from build123d import *

# Parameters (mm, degrees)
SKETCH1_R               = 12.7
BOSS_EXTRUDE1_DEPTH     = 0.79375
SKETCH2_R               = 9.525
BOSS_EXTRUDE2_DEPTH     = 6.35
SKETCH3_R               = 12.7
BOSS_EXTRUDE3_DEPTH     = 0.79375
SKETCH4_R               = 4.445
BOSS_EXTRUDE4_DEPTH     = 8.89
SKETCH5_R               = 3.175
CUT_EXTRUDE1_DEPTH      = 9.525
CUT_EXTRUDE2_DEPTH      = 25.4
CUT_EXTRUDE2_DEPTH_BACK = 25.4
SKETCH6_R               = 0.7874


with BuildPart() as part:
    # Sketch1 → Boss-Extrude1 (new body)
    with BuildSketch(Plane.XY):
        Circle(SKETCH1_R)
    extrude(amount=BOSS_EXTRUDE1_DEPTH)

    # Sketch2 → Boss-Extrude2 (add)
    with BuildSketch(Plane.XY.offset(0.79375)):
        Circle(SKETCH2_R)
    extrude(amount=BOSS_EXTRUDE2_DEPTH)

    # Sketch3 → Boss-Extrude3 (add)
    with BuildSketch(Plane.XY.offset(7.14375)):
        Circle(SKETCH3_R)
    extrude(amount=BOSS_EXTRUDE3_DEPTH)

    # Sketch4 → Boss-Extrude4 (add)
    with BuildSketch(Plane(origin=(0, 0, 0), x_dir=(-1, 0, 0), z_dir=(0, 0, -1))):
        Circle(SKETCH4_R)
    extrude(amount=BOSS_EXTRUDE4_DEPTH)

    # Sketch5 → Cut-Extrude1 (cut)
    with BuildSketch(Plane(origin=(0, 0, -8.89), x_dir=(-1, 0, 0), z_dir=(0, 0, -1))):
        Circle(SKETCH5_R)
    extrude(amount=-CUT_EXTRUDE1_DEPTH, mode=Mode.SUBTRACT)

    # Sketch6 → Cut-Extrude2 (cut, two sides: drawn at the far end of the back side and taken through both)
    with BuildSketch(Plane(origin=(0, 0, 0), x_dir=(1, 0, 0), z_dir=(0, 1, 0)).offset(-CUT_EXTRUDE2_DEPTH_BACK)):
        with Locations(Location((0, 5.715, 0), (0, 0, 90))):
            Circle(SKETCH6_R)
    extrude(amount=CUT_EXTRUDE2_DEPTH + CUT_EXTRUDE2_DEPTH_BACK, mode=Mode.SUBTRACT)


solid = part.part
Source: CAD feature listing. Evaluate the final solid. Frame: model axes, mm. A direction names the side the tool comes from. Give positions to 0.01 mm unless a question says otherwise; leave off trailing zeros. Write each loop counter-clockwise with the first axis right and the second up, starting at its lowest first coordinate (ties: lowest second). Pieces come first, ordered by that corner, then holes. Notation, with made-up numbers: M -14.75,84 L -2.75,84 A14 ccw -2.75,102 Z; hole C 63,18.25 d6. An arc over 180 degrees is marked long. Return JSON: item names as keys, results as strings. Group by question number.
1) Set-up query: faces 1 (the face through (5, 9, 7.144)), 2 (the face through (-2.75, -12.4, 0.39)), 3 (the face through (0, 0, 0.635)). Return all of +Z, -Z, +X, -X, +Y, -Y with unobstructed straight access to the full face (end or side cutting, diameter ignored); none if empty.
2) Cut plane B-B, the plane z = -4.25. Output: boundary loops of the cut face in (x, y) (3 decimals).
3) Cut plane A-A, the plane x = 0. Output: boundary loops of the cut face in (y, z) (1 decimal).
4) Cut plane C-C, the plane y = -3.5. Output: boundary loops of the cut face in (x, z) (1 decimal), then the cut area to 3 significant figures.
5) Ray query, L1, parallel to Z at x = 1.25, y = 11.75; L2, parallel to Y at x = 0, z = -3 (3 decimals); L3, parallel to Z at x = 3.5, y = 8.75. Return the intervals inside material, ascending.
6) Draft query along Z for faces 4 (the face through (0.302, -3.77, -6.442)), 5 (the face through (0, 0, 7.938)), 6 (the face through (-2, -3, -8.89)). Return one class per face: released by +Z, released by -Z, zero draft, split by the parting line, or undercut.
7) First-contact query: pin 1 Ø10 at (y, z) = (8, -5.5) entering from +X; pin 2 Ø1.8 at (x, z) = (0, -5.715) entering from +Y (3 decimals); pin 3 Ø3 at (y, z) = (-9, 3.5) entering from -X; pin 4 Ø0.9 at (x, z) = (0, -5.715) entering from -Y. Flat tips, straight axial feed; report the tip coordinate or a pass-through.
8) Cut plane D-D, the plane x = 10.75. Output: boundary loops of the cut face in (y, z), then the cut area to 3 significant figures.
Data:
{
 "1": {"face 1": "none", "face 2": "+Z, -Z", "face 3": "-Z"},
 "2": {"outline": "C 0,0 d8.89; hole C 0,0 d6.35"},
 "3": {"outline": "M -12.7,0 L -4.4,0 L -4.4,-4.9 L -3.2,-4.9 L -3.2,0.6 L 3.2,0.6 L 3.2,-4.9 L 4.4,-4.9 L 4.4,0 L 12.7,0 L 12.7,0.8 L 9.5,0.8 L 9.5,7.1 L 12.7,7.1 L 12.7,7.9 L -12.7,7.9 L -12.7,7.1 L -9.5,7.1 L -9.5,0.8 L -12.7,0.8 Z; M -4.4,-8.9 L -3.2,-8.9 L -3.2,-6.5 L -4.4,-6.5 Z; M 3.2,-8.9 L 4.4,-8.9 L 4.4,-6.5 L 3.2,-6.5 Z"},
 "4": {"outline": "M -12.2,0 L -2.7,0 L -2.7,-8.9 L 2.7,-8.9 L 2.7,0 L 12.2,0 L 12.2,0.8 L 8.9,0.8 L 8.9,7.1 L 12.2,7.1 L 12.2,7.9 L -12.2,7.9 L -12.2,7.1 L -8.9,7.1 L -8.9,0.8 L -12.2,0.8 Z; hole C 0,-5.7 d1.6", "area": "198 mm²"},
 "5": {"L1": "z = 0 to 0.79, 7.14 to 7.94", "L2": "y = -4.445 to -3.175, 3.175 to 4.445", "L3": "z = 0 to 7.94"},
 "6": {"face 4": "undercut", "face 5": "released by +Z", "face 6": "released by -Z"},
 "7": {"pin 1": "stops at x = 3.28", "pin 2": "stops at y = 4.445", "pin 3": "stops at x = -5.87", "pin 4": "passes through"},
 "8": {"outline": "M -6.76,0 L 6.76,0 L 6.76,0.79 L -6.76,0.79 Z; M -6.76,7.14 L 6.76,7.14 L 6.76,7.94 L -6.76,7.94 Z", "area": "21.5 mm²"}
}
